For this review, use the dimensioned drawing (mm, ordinates from the lowest corner) and the shaded views. A direction names the side the tool comes from. Give positions to 0.01 mm unless a question says otherwise; leave off trailing zeros. Write each loop counter-clockwise with the first axis right and the second up, starting at its lowest first coordinate (ties: lowest second). Pieces come first, ordered by that corner, then holes. Notation, with made-up numbers: (58.5, -30) -> (81.5, -30) arc R5 ccw to (81.5, -24) -> close; hole circle Ø9 at (89, 75). An arc over 180 degrees is marked (long way). Write each question's results on one line, items separated by ' | '. Start each with the question number.
(1) Take a section at A-A (y = 9.5). State the section outline as (x, z) points.
(2) Take a section at C-C (x = 25). State the section outline as (y, z) points.
(3) For the marked faces 1 and 2, list the 3-axis set-ups (+Z, -Z, +X, -X, +Y, -Y) from which the entire face can be reached by the end or side of a thin tool; tool diameter is ignored.
(4) Clearance check with a flat-ended pin moving along its axis: pin 1 (1 mm diameter, centred on x = 35, z = 6, fed in from +Y). State where the tip first meets the part, or that it passes through.
(5) To check wall thickness, follow probe 1 along Y at (x, z) = (47.5, 7.5). State the ranges of the line that lie inside material, in increasing order.
(6) Take a section at B-B (z = 7). State the section outline as (x, y) points, plus the area to 3 significant figures.
(7) Mouldability with a two-part tool opening along X and no side actions: class the marked faces 3, 4, 5 and 6 as released by +X, released by -X, zero draft, split by the parting line, or undercut.
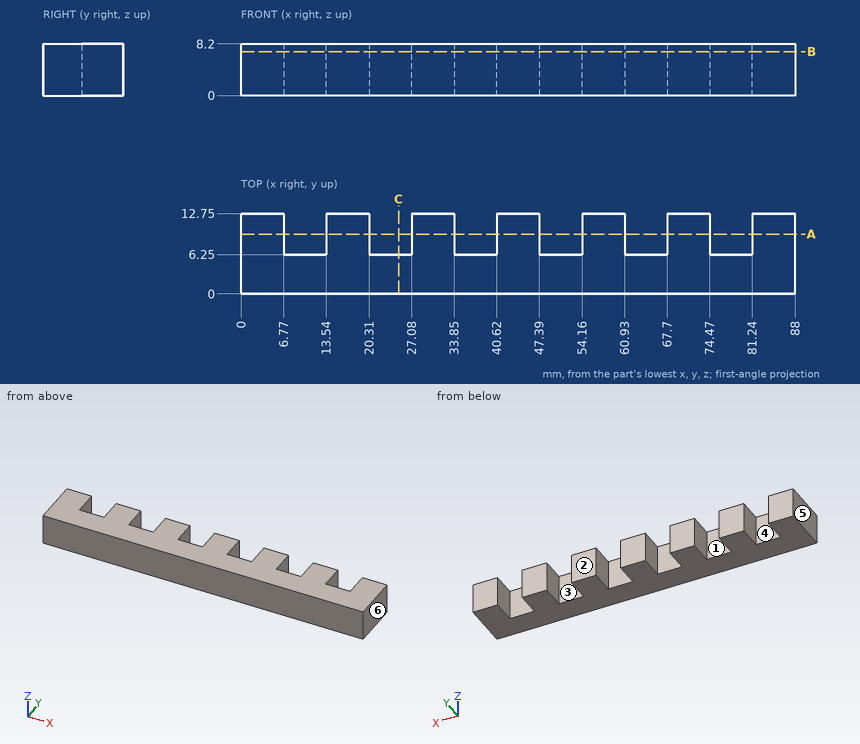
Report:
1) outline: (0, 0) -> (6.77, 0) -> (6.77, 8.2) -> (0, 8.2) -> close; (13.54, 0) -> (20.31, 0) -> (20.31, 8.2) -> (13.54, 8.2) -> close; (27.08, 0) -> (33.85, 0) -> (33.85, 8.2) -> (27.08, 8.2) -> close; (40.62, 0) -> (47.39, 0) -> (47.39, 8.2) -> (40.62, 8.2) -> close; (54.16, 0) -> (60.93, 0) -> (60.93, 8.2) -> (54.16, 8.2) -> close; (67.7, 0) -> (74.47, 0) -> (74.47, 8.2) -> (67.7, 8.2) -> close; (81.24, 0) -> (88, 0) -> (88, 8.2) -> (81.24, 8.2) -> close
2) outline: (0, 0) -> (6.25, 0) -> (6.25, 8.2) -> (0, 8.2) -> close
3) face 1: +Z, -Z, +Y | face 2: +Z, -Z, +X, -X, +Y
4) pin 1: y = 6.25
5) probe 1: 0 to 6.25
6) outline: (0, 0) -> (88, 0) -> (88, 12.75) -> (81.24, 12.75) -> (81.24, 6.25) -> (74.47, 6.25) -> (74.47, 12.75) -> (67.7, 12.75) -> (67.7, 6.25) -> (60.93, 6.25) -> (60.93, 12.75) -> (54.16, 12.75) -> (54.16, 6.25) -> (47.39, 6.25) -> (47.39, 12.75) -> (40.62, 12.75) -> (40.62, 6.25) -> (33.85, 6.25) -> (33.85, 12.75) -> (27.08, 12.75) -> (27.08, 6.25) -> (20.31, 6.25) -> (20.31, 12.75) -> (13.54, 12.75) -> (13.54, 6.25) -> (6.77, 6.25) -> (6.77, 12.75) -> (0, 12.75) -> close | area: 858 mm2
7) face 3: undercut | face 4: undercut | face 5: released by -X | face 6: released by +X
